Geometry: final body of the model. Coordinates: model frame, mm. A direction names the side the tool comes from. Round coordinates to 2 decimals unless told otherwise and drop trailing zeros. Write each loop counter-clockwise with the first axis right and the second up, starting at its lowest first coordinate (ties: lowest second). Pieces come first, ordered by that corner, then holes. Notation, with made-up numbers: M 3.5,36.5 L 21.5,36.5 A23 cw 21.5,47.5 Z; hole C 24.5,82 d5. An arc over 180 degrees is marked long. Answer as CSV lines item,"result". Start each with the question number.
Q1. Section query D-D on z = 17. Give the number of separate pieces and of enclosed holes in the cut face, and give its area (3 significant figures).
Q2. First-contact query: pin 1 (7.5 mm diameter, centred on x = 214.5, y = 0, fed in from +Z); pin 2 (8 mm diameter, centred on x = 152, y = 157, fed in from +Z); pin 3 (4 mm diameter, centred on y = 78, z = 25, fed in from +X); pin 4 (25 mm diameter, centred on x = 0, y = 214.5, fed in from -Z). Flat tips, straight axial feed; report the tip coordinate or a pass-through.
Q3. Ray query, probe 1 along X at (y, z) = (10.5, 31); probe 2 along Y at (x, z) = (-173, 4.5); probe 3 along X at (y, z) = (12.5, 2). Return the intervals inside material, ascending.
Q4. Section query A-A on x = 0. Output: boundary loops of the cut face in (y, z).
Q5. Mould query, pull axis X, two halves, no side actions, for faces 1 (the flat face through (34, 192, 38)), 2 (the cylindrical face through (31.18, 237.46, 4.44)), 3 (the cylindrical face through (2.981, -201.077, 32.577)), 4 (the flat face through (-2.9, -208.6, 27)). Classes: pulls with the +X half, pulls with the -X half, needs draft (parallel to the pull), parting line crosses it, or undercut.
Q6. Section query C-C on y = 214.5. Output: boundary loops of the cut face in (x, z).
Q7. Reachability of faces 5 (the flat face through (2.9, 208.6, 27)), 6 (the cylindrical face through (-2.884, -208.955, 13.689)) from +Z, -Z, +X, -X, +Y, -Y: full face, straight path, thin tool, end or side. Return the list, or none.
Autodesk Inventor part; units mm, degrees
ref_plane "YZ Plane" through (0, 0, 0) normal (1, 0, 0) x (0, 1, 0)
ref_plane "XZ Plane" through (0, 0, 0) normal (0, 1, 0) x (-1, 0, 0)
ref_plane "XY Plane" through (0, 0, 0) normal (0, 0, 1) x (1, 0, 0)
sketch "Sketch1" plane through (0, 0, 0) normal (0, 0, 1) x (1, 0, 0)
  circle A0 centre (0, 0) radius 194.5
  circle A1 centre (0, 0) radius 234.5
  dimension "d0" = 40
  dimension "d1" = 389
extrude "Extrusion1" add sketch "Sketch1" along normal blind 38
sketch "Sketch2" plane through (0, 0, 38) normal (0, 0, 1) x (1, 0, 0)
  circle A0 centre (0, 0) radius 234.5 construction
  circle A1 centre (0, 0) radius 194.5 construction
  line L0 (0, 234.5) -> (0, 194.5) construction
  circle A2 centre (0, 214.5) radius 6.25
  dimension "d4" = 12.5
extrude "Extrusion2" cut sketch "Sketch2" against normal through all
sketch "Sketch3" plane through (0, 0, 38) normal (0, 0, 1) x (1, 0, 0)
  circle A0 centre (0, 214.5) radius 6.25
  circle A1 centre (0, 214.5) radius 13.75
  point P0 (0, 0)
  dimension "d10" = 27.5
extrude "Extrusion3" cut sketch "Sketch3" against normal blind 11
pattern_circular "Circular Pattern1" count 8 over 360 about axis through (0, 0, 0) along (0, 0, 1) of "Extrusion2", "Extrusion3"
sketch "Sketch4" plane through (0, 0, 0) normal (0, 0, -1) x (-1, 0, 0)
  circle A0 centre (0, 0) radius 234.5
  circle A1 centre (0, 0) radius 239.5
  dimension "d13" = 5
extrude "Extrusion4" add sketch "Sketch4" against normal blind 9
equation "\"d1\" = Вал_ось_диаметр_КОРМА"
properties part number "ДМФ 01 32 Барабан Опорное кольцо КОРМА"
Entries:
1,separate pieces,"1"
1,enclosed holes,"9"
1,area,"52,900 mm^2"
2,pin 1,"passes through"
2,pin 2,"stops at z = 27"
2,pin 3,"stops at x = 221.84"
2,pin 4,"stops at z = 0"
3,probe 1,"x = -234.26 to -223.38, -205.62 to -194.22, 194.22 to 205.62, 223.38 to 234.26"
3,probe 2,"y = -165.62 to -88.89, 88.89 to 165.62"
3,probe 3,"x = -239.17 to -194.1, 194.1 to 239.17"
4,outline,"M -239.5,0 L -220.75,0 L -220.75,27 L -228.25,27 L -228.25,38 L -234.5,38 L -234.5,9 L -239.5,9 Z; M -208.25,0 L -194.5,0 L -194.5,38 L -200.75,38 L -200.75,27 L -208.25,27 Z; M 194.5,0 L 208.25,0 L 208.25,27 L 200.75,27 L 200.75,38 L 194.5,38 Z; M 220.75,0 L 239.5,0 L 239.5,9 L 234.5,9 L 234.5,38 L 228.25,38 L 228.25,27 L 220.75,27 Z"
5,face 1,"needs draft"
5,face 2,"parting line crosses it"
5,face 3,"undercut"
5,face 4,"undercut"
6,outline,"M -106.54,0 L -6.25,0 L -6.25,27 L -13.75,27 L -13.75,38 L -94.76,38 L -94.76,9 L -106.54,9 Z; M 6.25,0 L 106.54,0 L 106.54,9 L 94.76,9 L 94.76,38 L 13.75,38 L 13.75,27 L 6.25,27 Z"
7,face 5,"+Z"
7,face 6,"+Z, -Z"
